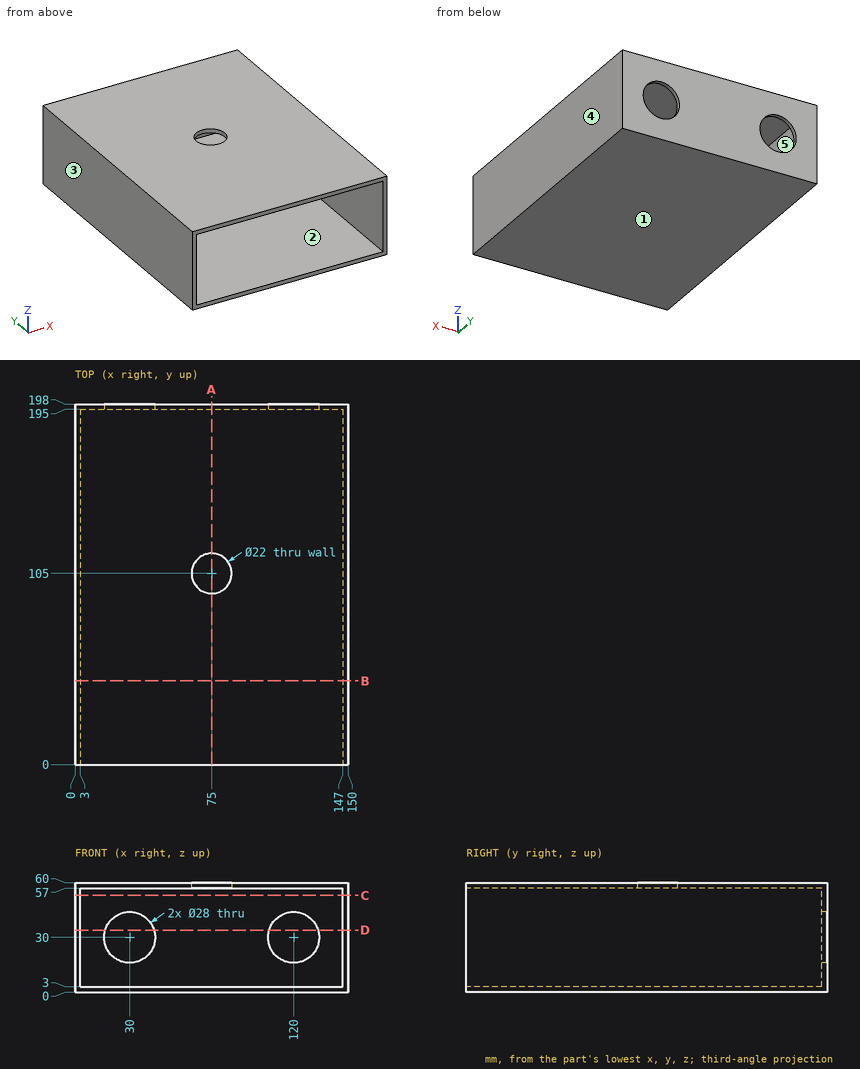
Geometry: see drawing. Coordinates: mm, zero at the bounding-box minimum. A direction names the side the tool comes from. Round coordinates to 2 decimals unless told otherwise and drop trailing zeros. Write each loop counter-clockwise with the first axis right and the second up, starting at its lowest first coordinate (ties: lowest second). Pieces come first, ordered by that corner, then holes. Notation, with made-up numbers: M 16.5,69 L 56.5,69 A14 ccw 56.5,79 Z; hole C -9.75,-24 d4. An arc over 180 degrees is marked long. Answer in a Markdown table with one row per item. Add a question column.
(1) Ray query, L1, parallel to Z at x = 120, y = 196.1; L2, parallel to Z at x = 61, y = 89; L3, parallel to X at y = 37, z = 18. Return the intervals inside material, ascending.
(2) Cut plane B-B, the plane y = 46. Return the cut outline in (x, z).
(3) Draft query along X for the marked faces 1, 2 and 3. Return one class per face: pulls with the +X half, pulls with the -X half, needs draft (parallel to the pull), parting line crosses it, or undercut.
(4) Cut plane C-C, the plane z = 53. Return the cut outline in (x, y), then the cut area to 3 significant figures.
(5) Reachability of the marked faces 4 and 5 from +Z, -Z, +X, -X, +Y, -Y: full face, straight path, thin tool, end or side. Return the list, or none.
(6) Contact query for flat-ended pins moving along their axis: pin 1 (13 mm diameter, centred on x = 75, y = 105, fed in from +Z); pin 2 (4 mm diameter, centred on x = 35, z = 53.5, fed in from -Y). Output: stop coordinate, or through.
(7) Cut plane A-A, the plane x = 75. Return the cut outline in (y, z), then the cut area to 3 significant figures.
(8) Cut plane D-D, the plane z = 34. Return the cut outline in (x, y), then the cut area to 3 significant figures.
Established:
| question | item | result |
|---|---|---|
| 1 | L1 | 0 to 16, 44 to 60 |
| 1 | L2 | 0 to 3, 57 to 60 |
| 1 | L3 | 0 to 3, 147 to 150 |
| 2 | outline | M 0,0 L 150,0 L 150,60 L 0,60 Z; hole M 3,3 L 147,3 L 147,57 L 3,57 Z |
| 3 | face 1 | needs draft |
| 3 | face 2 | undercut |
| 3 | face 3 | pulls with the -X half |
| 4 | outline | M 0,0 L 3,0 L 3,195 L 147,195 L 147,0 L 150,0 L 150,198 L 0,198 Z |
| 4 | area | 1,620 mm² |
| 5 | face 4 | +Z, -Z, +X, +Y, -Y |
| 5 | face 5 | -Y |
| 6 | pin 1 | z = 3 |
| 6 | pin 2 | y = 195 |
| 7 | outline | M 0,0 L 198,0 L 198,60 L 116,60 L 116,57 L 195,57 L 195,3 L 0,3 Z; M 0,57 L 94,57 L 94,60 L 0,60 Z |
| 7 | area | 1,280 mm² |
| 8 | outline | M 0,0 L 3,0 L 3,195 L 16.58,195 L 16.58,198 L 0,198 Z; M 43.42,195 L 106.58,195 L 106.58,198 L 43.42,198 Z; M 133.42,195 L 147,195 L 147,0 L 150,0 L 150,198 L 133.42,198 Z |
| 8 | area | 1,460 mm² |
